Source: CAD feature listing. Evaluate the final solid. Frame: model axes, mm. A direction names the side the tool comes from. Round coordinates to 2 decimals unless told otherwise and drop trailing zeros. Write each loop counter-clockwise with the first axis right and the second up, starting at its lowest first coordinate (ties: lowest second). Pieces come first, ordered by that corner, then holes. Notation, with made-up numbers: M 14,-3.75 L 73,-3.75 A17 ccw 73,28.25 Z; hole C -30,-31 d7. An arc over 180 degrees is marked long. Answer in a Markdown table with one row per item. Add a question column.
Item 1: Set-up query: faces 5 (the face through (4.201, -18, 5)), 6 (the face through (0, -10, 3)), 7 (the face through (-14, 0, 3)). Return all of +Z, -Z, +X, -X, +Y, -Y with unobstructed straight access to the full face (end or side cutting, diameter ignored); none if empty.
Item 2: Cut plane D-D on y = -11. Return loops of the section in (x, z), and give its area (3 significant figures).
Item 3: Cut plane A-A on y = 14.5. Return loops of the section in (x, z).
Item 4: Cut plane C-C on z = 4.25. Return loops of the section in (x, y), and give its area (3 significant figures).
Item 5: Mould query, pull axis Y, two halves, no side actions, for faces 1 (the face through (20.458, 6.535, 1.085)), 2 (the face through (10.29, -16.48, 1.08)), 3 (the face through (-12, -3.75, 3)), 4 (the face through (0, 20, 3.7)). Classes: released by +Y, released by -Y, zero draft, split by the parting line, or undercut.
Item 6: Contact query for flat-ended pins moving along their axis: pin 1 (6 mm diameter, centred on x = -6.5, y = 6.5, fed in from +Z); pin 2 (4.5 mm diameter, centred on x = -12.5, y = -1.5, fed in from +Z); pin 3 (6 mm diameter, centred on x = -1, y = 20, fed in from +Z). Output: stop coordinate, or through.
Item 7: Material intervals for probe 1 along Y at (x, z) = (-8, 1.5); probe 2 along X at (y, z) = (-17, 1.25); probe 3 along X at (y, z) = (14.5, 1.25), sorted ascending.
Item 8: Cut plane B-B on x = 15. Return loops of the section in (y, z).
from build123d import *

# Parameters (mm, degrees)
F0_R     = 1.65
F0_W     = 3.56
F0_H     = 3
F0_W_2   = 5
F0_H_2   = 5
F0_W_3   = 4
F0_H_3   = 7.5
F1_DEPTH = 2.2
F2_DEPTH = 3.7
F3_DEPTH = 7
F4_DEPTH = 3.6
F5_DEPTH = 2.5
F6_DEPTH = 3


with BuildPart() as f1:
    # F0 (on Top) → F1 (new body)
    with BuildSketch(Plane.XY):
        with BuildLine():
            ThreePointArc((4.20097, -22.10434), (17.331645, -14.347965), (22.5, 0))
            ThreePointArc((22.5, 0), (17.266613, 14.42616), (4.00097, 22.141415))
            Line((4.00097, 22.141415), (4.00097, 16.75))
            Line((4.00097, 16.75), (-3.99903, 16.75))
            Line((-3.99903, 16.75), (-3.99903, 22.141765))
            ThreePointArc((-3.99903, 22.141765), (-22.5, 0), (-3.99903, -22.141765))
            Line((-3.99903, -22.141765), (-3.99903, -14.35))
            Line((-3.99903, -14.35), (4.20097, -14.35))
            Line((4.20097, -14.35), (4.20097, -22.10434))
        make_face()
        with Locations((-15.153525, -13.395359)):
            Circle(F0_R, mode=Mode.SUBTRACT)
        with Locations((-9.405204, -17.872991)):
            Circle(F0_R, mode=Mode.SUBTRACT)
        with Locations((-18.933541, -7.166085)):
            Circle(F0_R, mode=Mode.SUBTRACT)
        with Locations((9.405204, -17.872991)):
            Circle(F0_R, mode=Mode.SUBTRACT)
        with Locations((15.153525, -13.395359)):
            Circle(F0_R, mode=Mode.SUBTRACT)
        with Locations((0, -10.25)):
            Rectangle(F0_W, F0_H, mode=Mode.SUBTRACT)
        with Locations((0, -6)):
            Rectangle(F0_W_2, F0_H_2, mode=Mode.SUBTRACT)
        with Locations((18.933541, -7.166085)):
            Circle(F0_R, mode=Mode.SUBTRACT)
        with Locations((-20.25097, 0.000278)):
            Circle(F0_R, mode=Mode.SUBTRACT)
        with Locations((-12, 0)):
            Rectangle(F0_W_3, F0_H_3, mode=Mode.SUBTRACT)
        with Locations((-18.933541, 7.166641)):
            Circle(F0_R, mode=Mode.SUBTRACT)
        with Locations((-15.153525, 13.395914)):
            Circle(F0_R, mode=Mode.SUBTRACT)
        with Locations((-9.405204, 17.873546)):
            Circle(F0_R, mode=Mode.SUBTRACT)
        with Locations((20.25097, 0.000278)):
            Circle(F0_R, mode=Mode.SUBTRACT)
        with Locations((18.933541, 7.166641)):
            Circle(F0_R, mode=Mode.SUBTRACT)
        with Locations((9.405204, 17.873546)):
            Circle(F0_R, mode=Mode.SUBTRACT)
        with Locations((15.153525, 13.395914)):
            Circle(F0_R, mode=Mode.SUBTRACT)
    extrude(amount=F1_DEPTH)

    # F0 (on Top) → F2 (join)
    with BuildSketch(Plane.XY):
        with BuildLine():
            Line((4.00097, 16.75), (4.00097, 22.141415))
            ThreePointArc((4.00097, 22.141415), (3.673272, 22.198132), (3.344772, 22.25))
            Line((3.344772, 22.25), (-3.344772, 22.25))
            ThreePointArc((-3.344772, 22.25), (-3.6723, 22.198293), (-3.99903, 22.141765))
            Line((-3.99903, 22.141765), (-3.99903, 16.75))
            Line((-3.99903, 16.75), (4.00097, 16.75))
        make_face()
    extrude(amount=F2_DEPTH)

    # F0 (on Top) → F3 (join)
    with BuildSketch(Plane.XY):
        with BuildLine():
            ThreePointArc((2.593742, -22.35), (3.399576, -22.241692), (4.20097, -22.10434))
            Line((4.20097, -22.10434), (4.20097, -14.35))
            Line((4.20097, -14.35), (-3.99903, -14.35))
            Line((-3.99903, -14.35), (-3.99903, -22.141765))
            ThreePointArc((-3.99903, -22.141765), (-3.29803, -22.256976), (-2.593742, -22.35))
            Line((-2.593742, -22.35), (2.593742, -22.35))
        make_face()
    extrude(amount=F3_DEPTH)

    # F0 (on Top) → F4 (join)
    with BuildSketch(Plane.XY):
        with Locations((-12, 0)):
            Rectangle(F0_W_3, F0_H_3)
    extrude(amount=F4_DEPTH)

    # F0 (on Top) → F5 (join)
    with BuildSketch(Plane.XY):
        with Locations((0, -6)):
            Rectangle(F0_W_2, F0_H_2)
    extrude(amount=F5_DEPTH)

    # F0 (on Top) → F6 (join)
    with BuildSketch(Plane.XY):
        with Locations((0, -10.25)):
            Rectangle(F0_W, F0_H)
    extrude(amount=F6_DEPTH)


solid = f1.part
Results below:
| question | item | result |
|---|---|---|
| 1 | face 5 | +Z, +X, +Y, -Y |
| 1 | face 6 | +Z, +X, -X |
| 1 | face 7 | +Z, -X, +Y, -Y |
| 2 | outline | M -19.63,0 L 19.63,0 L 19.63,2.2 L 1.78,2.2 L 1.78,3 L -1.78,3 L -1.78,2.2 L -19.63,2.2 Z |
| 2 | area | 89.2 mm2 |
| 3 | outline | M -17.2,0 L -16.38,0 L -16.38,2.2 L -17.2,2.2 Z; M -13.93,0 L 13.93,0 L 13.93,2.2 L -13.93,2.2 Z; M 16.38,0 L 17.2,0 L 17.2,2.2 L 16.38,2.2 Z |
| 4 | outline | M -4,-22.14 A22.5 ccw -2.59,-22.35 L 2.59,-22.35 A22.5 ccw 4.2,-22.1 L 4.2,-14.35 L -4,-14.35 Z |
| 4 | area | 65.3 mm2 |
| 5 | face 1 | undercut |
| 5 | face 2 | undercut |
| 5 | face 3 | released by -Y |
| 5 | face 4 | zero draft |
| 6 | pin 1 | z = 2.2 |
| 6 | pin 2 | z = 3.6 |
| 6 | pin 3 | z = 3.7 |
| 7 | probe 1 | -21.03 to -18.74, -17.01 to 17.01, 18.74 to 21.03 |
| 7 | probe 2 | -14.74 to -10.81, -8.01 to 8.01, 10.81 to 14.74 |
| 7 | probe 3 | -17.2 to -16.38, -13.93 to 13.93, 16.38 to 17.2 |
| 8 | outline | M -16.77,0 L -15.04,0 L -15.04,2.2 L -16.77,2.2 Z; M -11.75,0 L 11.75,0 L 11.75,2.2 L -11.75,2.2 Z; M 15.04,0 L 16.77,0 L 16.77,2.2 L 15.04,2.2 Z |
